from build123d import *

# Parameters (mm, degrees)
F1_DEPTH = 3
F3_DEPTH = 3.001
F5_D     = 6.6


with BuildPart() as f1:
    # F0 (on Front) → F1 (new body)
    with BuildSketch(Plane.XZ):
        Polygon((-249.1925892383, 121.4087251365), (-249.1925892383, -132.5912748635), (-198.3925892383, -30.9912748635), (208.0074107617, -30.9912748635), (258.8074107617, -132.5912748635), (258.8074107617, 121.4087251365), (208.0074107617, 223.0087251365), (-198.3925892383, 223.0087251365), align=None)
    extrude(amount=F1_DEPTH)

    # F2 (on face) → F3 (cut, through all)
    with BuildSketch(Plane.XZ.offset(3)):
        with BuildLine():
            ThreePointArc((-198.3925892383, 45.2087251365), (-190.9531014804, 27.2482128944), (-172.9925892383, 19.8087251365))
            Line((-172.9925892383, 19.8087251365), (-71.3925892383, 19.8087251365))
            ThreePointArc((-71.3925892383, 19.8087251365), (-53.4320769961, 27.2482128944), (-45.9925892383, 45.2087251365))
            Line((-45.9925892383, 45.2087251365), (-45.9925892383, 146.8087251365))
            ThreePointArc((-45.9925892383, 146.8087251365), (-53.4320769961, 164.7692373787), (-71.3925892383, 172.2087251365))
            Line((-71.3925892383, 172.2087251365), (-151.2983992955, 172.2087251365))
            ThreePointArc((-151.2983992955, 172.2087251365), (-164.6519695434, 168.4152556687), (-174.0168499469, 158.1679504622))
            Line((-174.0168499469, 158.1679504622), (-195.7110398897, 114.7795705767))
            ThreePointArc((-195.7110398897, 114.7795705767), (-197.7131135708, 109.2560694329), (-198.3925892383, 103.420345251))
            Line((-198.3925892383, 103.420345251), (-198.3925892383, 45.2087251365))
        make_face()
        with BuildLine():
            ThreePointArc((208.0074107617, 103.420345251), (207.3279350942, 109.2560694329), (205.3258614131, 114.7795705767))
            Line((205.3258614131, 114.7795705767), (183.6316714704, 158.1679504622))
            ThreePointArc((183.6316714704, 158.1679504622), (174.2667910668, 168.4152556687), (160.913220819, 172.2087251365))
            Line((160.913220819, 172.2087251365), (81.0074107617, 172.2087251365))
            ThreePointArc((81.0074107617, 172.2087251365), (63.0468985196, 164.7692373787), (55.6074107617, 146.8087251365))
            Line((55.6074107617, 146.8087251365), (55.6074107617, 45.2087251365))
            ThreePointArc((55.6074107617, 45.2087251365), (63.0468985196, 27.2482128944), (81.0074107617, 19.8087251365))
            Line((81.0074107617, 19.8087251365), (182.6074107617, 19.8087251365))
            ThreePointArc((182.6074107617, 19.8087251365), (200.5679230039, 27.2482128944), (208.0074107617, 45.2087251365))
            Line((208.0074107617, 45.2087251365), (208.0074107617, 103.420345251))
        make_face()
    extrude(amount=-F3_DEPTH, mode=Mode.SUBTRACT)

    # F5 (through all)
    with Locations(Plane.XZ.offset(3)):
        with Locations((-172.9925892383, 210.5087251365), (4.8074107617, 210.5087251365), (182.6074107617, 210.5087251365), (246.3074107617, 96.0087251365), (246.3074107617, -81.7912748635), (-236.6925892383, -81.7912748635), (-236.6925892383, 96.0087251365)):
            Hole(F5_D / 2)


solid = f1.part
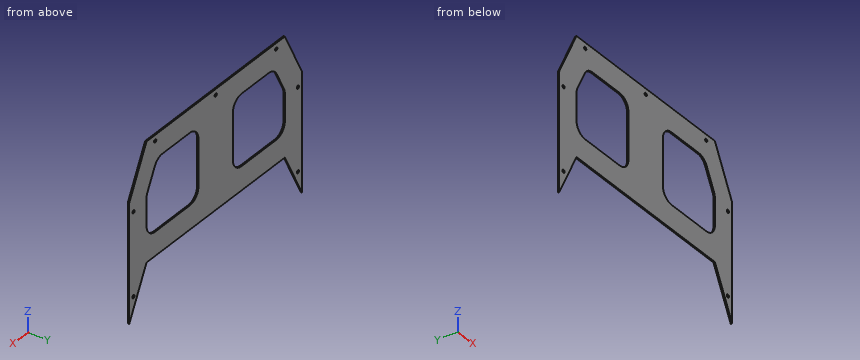
Build history of the part. All positions in model axes, mm. Round coordinates to 2 decimals unless told otherwise and drop trailing zeros. Write each loop counter-clockwise with the first axis right and the second up, starting at its lowest first coordinate (ties: lowest second). Pieces come first, ordered by that corner, then holes. Notation, with made-up numbers: (66, 24) - (70, 24) arc R32 cw to (70, 55) - close; hole circle Ø10 at (66.5, -11). An arc over 180 degrees is marked (long way). Use CSV: the item, a comma, the result in double quotes.
(1) Band-saw the part on C-C (x = 20). Write the cut outline in (y, z), plus the area to 3 significant figures.
Response:
outline,"(-3, -30.99) - (0, -30.99) - (0, 223.01) - (-3, 223.01) - close"
area,"762 mm²"
(2) Wall check: line 1 (X direction, y = -1.15, z = 55); line 2 (Z direction, x = -81, y = -1.65); line 3 (X direction, y = -0.9, z = 136.5). Give the ranges that are in metal, low to high.
Response:
line 1,"-249.19 to -198.39, -45.99 to 55.61, 208.01 to 258.81"
line 2,"-30.99 to 19.81, 172.21 to 223.01"
line 3,"-241.65 to -184.85, -45.99 to 55.61, 194.47 to 251.26"
(3) Band-saw the part on A-A (x = -106.5). Write the cut outline in (y, z), plus the area to 3 significant figures.
Response:
outline,"(-3, -30.99) - (0, -30.99) - (0, 19.81) - (-3, 19.81) - close; (-3, 172.21) - (0, 172.21) - (0, 223.01) - (-3, 223.01) - close"
area,"305 mm²"
(4) Band-saw the part on B-B (z = -68). Write the cut outline in (x, y).
Response:
outline,"(-249.19, -3) - (-216.9, -3) - (-216.9, 0) - (-249.19, 0) - close; (226.51, -3) - (258.81, -3) - (258.81, 0) - (226.51, 0) - close"
(5) Band-saw the part on D-D (y = -1.2). Give the number of separate pieces and of enclosed holes in the cut face, plus the area to 3 significant figures.
Response:
separate pieces,"1"
enclosed holes,"9"
area,"85,200 mm²"
(6) Pin check, flat tip, straight feed: P1, Ø1.5, axis at x = 110, y = -2, coming from the -Z side. Stop position of the tip, or through.
Response:
P1,"z = -30.99"
